Geometry: final body of the model. Coordinates: model frame, mm. Face numbers are marked on the shaded views. Round coordinates to 2 decimals unless told otherwise and drop trailing zeros. Loops run counter-clockwise (first coordinate to the right, second up) from the corner with the lowest first, then second, coordinate; pieces in that order, holes last. Notation, with made-up numbers: (40, 37) - (84, 37) arc R29 ccw to (84, 57) - close; hole circle Ø5 at (10, -31.75). An arc over 180 degrees is marked (long way). Use CSV: the item, a comma, the result in double quotes.
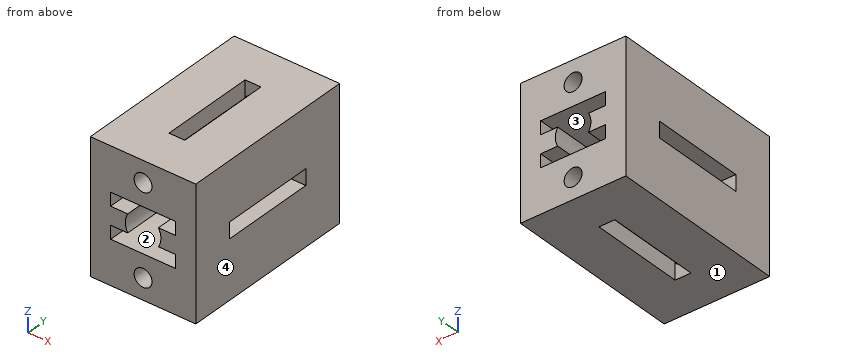
from build123d import *

# Parameters (mm, degrees)
F1_DEPTH = 17
F2_W     = 3
F2_H     = 18
F3_DEPTH = 25.001
F4_W     = 18
F4_H     = 3
F5_DEPTH = 20.001
F7_D     = 3.4
F7_DEPTH = 35
F7_TIP   = 1.0214630523


with BuildPart() as f1:
    # F0 (on Front) → F1 (new body, symmetric)
    with BuildSketch(Plane.XZ):
        with BuildLine():
            Line((-1.1521708115, 1.7021708115), (-1.1521708115, 4.2021708115))
            Line((-1.1521708115, 4.2021708115), (5, 4.2021708115))
            Line((5, 4.2021708115), (5, 12.5))
            Line((5, 12.5), (-5, 12.5))
            Line((-5, 12.5), (-5, -12.5))
            Line((-5, -12.5), (5, -12.5))
            Line((5, -12.5), (5, -4.2021708115))
            Line((5, -4.2021708115), (-1.1521708115, -4.2021708115))
            Line((-1.1521708115, -4.2021708115), (-1.1521708115, -1.7021708115))
            Line((-1.1521708115, -1.7021708115), (2.0856836945, -1.7021708115))
            ThreePointArc((2.0856836945, -1.7021708115), (1.625, 0), (2.0856836945, 1.7021708115))
            Line((2.0856836945, 1.7021708115), (-1.1521708115, 1.7021708115))
        make_face()
        with BuildLine():
            Line((5, 12.5), (5, 4.2021708115))
            Line((5, 4.2021708115), (11.1521708115, 4.2021708115))
            Line((11.1521708115, 4.2021708115), (11.1521708115, 1.7021708115))
            Line((11.1521708115, 1.7021708115), (7.9143163055, 1.7021708115))
            ThreePointArc((7.9143163055, 1.7021708115), (8.375, 0), (7.9143163055, -1.7021708115))
            Line((7.9143163055, -1.7021708115), (11.1521708115, -1.7021708115))
            Line((11.1521708115, -1.7021708115), (11.1521708115, -4.2021708115))
            Line((11.1521708115, -4.2021708115), (5, -4.2021708115))
            Line((5, -4.2021708115), (5, -12.5))
            Line((5, -12.5), (15, -12.5))
            Line((15, -12.5), (15, 12.5))
            Line((15, 12.5), (5, 12.5))
        make_face()
    extrude(amount=F1_DEPTH, both=True)

    # F2 (on face) → F3 (cut, through all)
    with BuildSketch(Plane.XY.offset(12.5)):
        with Locations((5, 0)):
            Rectangle(F2_W, F2_H)
    extrude(amount=-F3_DEPTH, mode=Mode.SUBTRACT)

    # F4 (on face) → F5 (cut, through all)
    with BuildSketch(Plane.YZ.offset(15)):
        Rectangle(F4_W, F4_H)
    extrude(amount=-F5_DEPTH, mode=Mode.SUBTRACT)

    # F7
    with Locations(Plane.XZ.offset(17)):
        with Locations((5, 8.5), (5, -8.5)):
            Hole(F7_D / 2, depth=F7_DEPTH)
            with Locations((0, 0, -(F7_DEPTH + F7_TIP / 2))):  # 118° drill point
                Cone(0, F7_D / 2, F7_TIP, mode=Mode.SUBTRACT)


solid = f1.part
Item 1: Section C-C on x = 5. Give the number of separate pieces and of enclosed holes in the cut face, plus the area to 3 significant figures.
Final values:
separate pieces,"8"
enclosed holes,"0"
area,"157 mm²"
Item 2: Material intervals for line 1 (Z direction, x = 10, y = 12.5); line 2 (Z direction, x = 8.5, y = 1); line 3 (Z direction, x = 6.5, y = 12.5), sorted ascending.
Final values:
line 1,"z = -12.5 to -4.2, -1.7 to 1.7, 4.2 to 12.5"
line 2,"z = -12.5 to -4.2, -1.7 to -1.5, 1.5 to 1.7, 4.2 to 12.5"
line 3,"z = -12.5 to -9.3, -7.7 to -4.2, 4.2 to 7.7, 9.3 to 12.5"
Item 3: Pin query (flat end, axial travel): P1, Ø2.5, axis at x = 5, z = -8.5, coming from the +Y side. Return the tip coordinate at first contact, or that it passes through.
Final values:
P1,"passes through"
Item 4: Section B-B on x = 1. Return the cut outline in (y, z), plus the area to 3 significant figures.
Final values:
outline,"(-17, -12.5) - (17, -12.5) - (17, -4.2) - (-17, -4.2) - close; (-17, -1.7) - (17, -1.7) - (17, 1.7) - (-17, 1.7) - close; (-17, 4.2) - (17, 4.2) - (17, 12.5) - (-17, 12.5) - close; hole (-9, -1.5) - (9, -1.5) - (9, 1.5) - (-9, 1.5) - close"
area,"626 mm²"
Item 5: Section A-A on z = 3.5. Return the cut outline in (x, y), plus the area to 3 significant figures.
Final values:
outline,"(-5, -17) - (-1.15, -17) - (-1.15, 17) - (-5, 17) - close; (11.15, -17) - (15, -17) - (15, 17) - (11.15, 17) - close"
area,"262 mm²"
Item 6: Section D-D on x = -2.25. Return the cut outline in (y, z), plus the area to 3 significant figures.
Final values:
outline,"(-17, -12.5) - (17, -12.5) - (17, 12.5) - (-17, 12.5) - close; hole (-9, -1.5) - (9, -1.5) - (9, 1.5) - (-9, 1.5) - close"
area,"796 mm²"
Item 7: Mould query, pull axis X, two halves, no side actions, for the marked faces 1, 2, 3 and 4. Classes: released by +X, released by -X, zero draft, split by the parting line, or undercut.
Final values:
face 1,"zero draft"
face 2,"undercut"
face 3,"undercut"
face 4,"released by +X"
